```python
from build123d import *

# Parameters (mm, degrees)
SKETCH_1_R               = 10
EXTRUDE_1_DEPTH          = 8
CUT_EXTRUDE_START        = -4
SKETCH_2_R               = 10
SKETCH_2_R_2             = 7.5
CUT_EXTRUDE_1_DEPTH      = 4
CUT_EXTRUDE_2_DEPTH      = 18.211914478
CUT_EXTRUDE_2_DEPTH_BACK = 18.211914478
SKETCH_3_R               = 1.3
SKETCH_4_R               = 0.75
CUT_EXTRUDE_3_DEPTH      = 4


with BuildPart() as part:
    # 草图1 → 凸台-拉伸1 (new body)
    with BuildSketch(Plane(origin=(0, 0, 0), x_dir=(1, 0, 0), z_dir=(0, 1, 0))):
        with Locations(Location((0, 0, 0), (0, 0, 270))):
            Circle(SKETCH_1_R)
        with BuildLine():
            Line((-1.5, 2), (-1.5, -2))
            ThreePointArc((-1.5, -2), (0, -2.5), (1.5, -2))
            Line((1.5, -2), (1.5, 2))
            ThreePointArc((1.5, 2), (0, 2.5), (-1.5, 2))
        make_face(mode=Mode.SUBTRACT)
    extrude(amount=EXTRUDE_1_DEPTH)

    # 草图2 → 切除-拉伸1 (cut)
    with BuildSketch(Plane(origin=(0, 8, 0), x_dir=(1, 0, 0), z_dir=(0, 1, 0)).offset(CUT_EXTRUDE_START)):
        with Locations(Location((0, 0, 0), (0, 0, 270))):
            Circle(SKETCH_2_R)
        with Locations(Location((0, 0, 0), (0, 0, 270))):
            Circle(SKETCH_2_R_2, mode=Mode.SUBTRACT)
    extrude(amount=CUT_EXTRUDE_1_DEPTH, mode=Mode.SUBTRACT)

    # 草图3 → 切除-拉伸2 (cut, two sides: drawn at the far end of the back side and taken through both)
    with BuildSketch(Plane(origin=(-1.5, 0, 0), x_dir=(0, 0, -1), z_dir=(1, 0, 0)).offset(-CUT_EXTRUDE_2_DEPTH_BACK)):
        with Locations(Location((0, 3, 0), (0, 0, 309.715229307))):
            Circle(SKETCH_3_R)
    extrude(amount=CUT_EXTRUDE_2_DEPTH + CUT_EXTRUDE_2_DEPTH_BACK, mode=Mode.SUBTRACT)

    # 草图4 → 切除-拉伸3 (cut)
    with BuildSketch(Plane(origin=(0, 4, 0), x_dir=(1, 0, 0), z_dir=(0, 1, 0))):
        with Locations(Location((-5.5, 5.5, 0), (0, 0, 270))):
            Circle(SKETCH_4_R)
        with Locations(Location((5.5, 5.5, 0), (0, 0, 270))):
            Circle(SKETCH_4_R)
        with Locations(Location((-5.5, -5.5, 0), (0, 0, 270))):
            Circle(SKETCH_4_R)
        with Locations(Location((5.5, -5.5, 0), (0, 0, 270))):
            Circle(SKETCH_4_R)
    extrude(amount=-CUT_EXTRUDE_3_DEPTH, mode=Mode.SUBTRACT)


solid = part.part
```
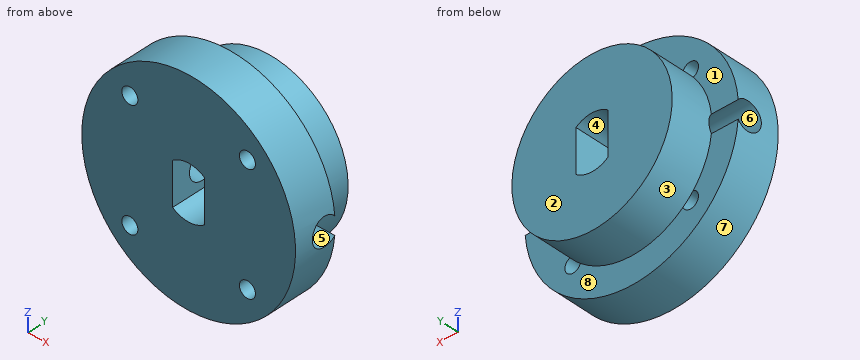
Source: CAD feature listing. Evaluate the final solid. Frame: model axes, mm. Face numbers are marked on the shaded views. A direction names the side the tool comes from. Coordinates: 2 decimals unless noted, no trailing zeros. Write each loop counter-clockwise with the first axis right and the second up, starting at its lowest first coordinate (ties: lowest second). Pieces come first, ordered by that corner, then holes. Notation, with made-up numbers: (78, -2) -> (113, -2) arc R30 ccw to (113, 20) -> close; hole circle Ø6 at (9.25, 53.25). An arc over 180 degrees is marked (long way). Return JSON: item names as keys, results as strings. Group by question number.
1) Section query C-C, the plane z = 0. Return loops of the section in (x, y), plus the area to 3 significant figures.
2) Mould query, pull axis Z, two halves, no side actions, for the marked faces 6, 7 and 8. Classes: +Z half, -Z half, draft (parallel to the pull), parting line (faces both ways), or undercut.
3) Contact query for flat-ended pins moving along their axis: P1, Ø1.7, axis at x = 5.5, z = 5.5, coming from the +Y side; P2, Ø3, axis at y = 3.5, z = 0, coming from the +X side; P3, Ø1, axis at y = 4, z = -1.5, coming from the -X side; P4, Ø3, axis at y = 3.5, z = -0.5, coming from the -X side. Output: stop coordinate, or through.
4) Section query A-A, the plane y = 3. Return loops of the section in (x, z), plus the area to 3 significant figures.
5) Ray query, line 1 along X through (y, z) = (1.6, 5.5); line 2 along Z through (x, y) = (-5.5, 2.85); line 3 along Z through (x, y) = (-6, 3). Return the intervals inside material, ascending.
6) Set-up query: the marked faces 1, 2, 3, 4 and 5. Return all of +Z, -Z, +X, -X, +Y, -Y with unobstructed straight access to the full face (end or side cutting, diameter ignored); none if empty.
7) Section query D-D, the plane z = 5.5. Return loops of the section in (x, y).
8) Section query B-B, the plane x = 5.5. Return loops of the section in (y, z).
From the geometry:
{
 "1": {"outline": "(-10, 0) -> (-1.5, 0) -> (-1.5, 1.7) -> (-10, 1.7) -> close; (-7.5, 4.3) -> (-1.5, 4.3) -> (-1.5, 8) -> (-7.5, 8) -> close; (1.5, 0) -> (10, 0) -> (10, 1.7) -> (1.5, 1.7) -> close; (1.5, 4.3) -> (7.5, 4.3) -> (7.5, 8) -> (1.5, 8) -> close", "area": "73.3 mm²"},
 "2": {"face 6": "undercut", "face 7": "parting line", "face 8": "draft"},
 "3": {"P1": "y = 8", "P2": "x = 9.97", "P3": "x = -9.95", "P4": "x = -9.97"},
 "4": {"outline": "(-9.92, -1.3) arc R10 ccw to (9.92, -1.3) -> (1.5, -1.3) -> (1.5, -2) arc R2.5 cw to (-1.5, -2) -> (-1.5, -1.3) -> close; (-9.92, 1.3) -> (-1.5, 1.3) -> (-1.5, 2) arc R2.5 cw to (1.5, 2) -> (1.5, 1.3) -> (9.92, 1.3) arc R10 ccw to start; hole circle Ø1.5 at (-5.5, -5.5); hole circle Ø1.5 at (-5.5, 5.5); hole circle Ø1.5 at (5.5, -5.5); hole circle Ø1.5 at (5.5, 5.5)", "area": "249 mm²"},
 "5": {"line 1": "-8.35 to -6.25, -4.75 to 4.75, 6.25 to 8.35", "line 2": "-8.35 to -6.25, -4.75 to -1.29, 1.29 to 4.75, 6.25 to 8.35", "line 3": "-8 to -6.06, -4.94 to -1.3, 1.3 to 4.94, 6.06 to 8"},
 "6": {"face 1": "+Z, +Y", "face 2": "+Z, -Z, +X, -X, +Y", "face 3": "+Y", "face 4": "+Y, -Y", "face 5": "+X, -X"},
 "7": {"outline": "(-8.35, 0) -> (-6.25, 0) -> (-6.25, 4) -> (-8.35, 4) -> close; (-5.1, 4) -> (-4.75, 4) -> (-4.75, 0) -> (4.75, 0) -> (4.75, 4) -> (5.1, 4) -> (5.1, 8) -> (-5.1, 8) -> close; (6.25, 0) -> (8.35, 0) -> (8.35, 4) -> (6.25, 4) -> close"},
 "8": {"outline": "(0, -8.35) -> (4, -8.35) -> (4, -6.25) -> (0, -6.25) -> close; (0, -4.75) -> (4, -4.75) -> (4, -5.1) -> (8, -5.1) -> (8, 5.1) -> (4, 5.1) -> (4, 4.75) -> (0, 4.75) -> close; (0, 6.25) -> (4, 6.25) -> (4, 8.35) -> (0, 8.35) -> close; hole circle Ø2.6 at (3, 0)"}
}
